```python
from build123d import *

# Parameters (mm, degrees)
SKETCH1_W           = 65
SKETCH1_H           = 68
BOSS_EXTRUDE1_DEPTH = 20
FILLET1_R           = 5
FILLET2_R           = 2
CUT_EXTRUDE1_DEPTH  = 2
FILLET3_R           = 0.5
SKETCH3_W           = 3
SKETCH3_H           = 3
BOSS_EXTRUDE2_DEPTH = 4
FILLET4_R           = 0.2


with BuildPart() as part:
    # Sketch1 → Boss-Extrude1 (new body)
    with BuildSketch(Plane(origin=(0, 0, 0), x_dir=(1, 0, 0), z_dir=(0, 1, 0))):
        Rectangle(SKETCH1_W, SKETCH1_H)
    extrude(amount=BOSS_EXTRUDE1_DEPTH)

    # Fillet1
    fillet1_edges = [part.edges().sort_by_distance(p)[0] for p in [
        (-32.5, 20, 0),
        (32.5, 20, 0),
        (-32.5, 0, 0),
        (32.5, 0, 0),
    ]]
    fillet(fillet1_edges, radius=FILLET1_R)

    # Fillet2
    fillet2_edges = [part.edges().sort_by_distance(p)[0] for p in [
        (-32.5, 10, 34),
        (-32.5, 10, -34),
        (0, 0, 34),
        (32.5, 10, 34),
        (0, 20, 34),
        (31.035533906, 18.535533906, 34),
        (31.035533906, 1.464466094, 34),
        (-31.035533906, 18.535533906, 34),
        (-31.035533906, 1.464466094, 34),
        (0, 0, -34),
        (0, 20, -34),
        (32.5, 10, -34),
        (31.035533906, 18.535533906, -34),
        (31.035533906, 1.464466094, -34),
        (-31.035533906, 18.535533906, -34),
        (-31.035533906, 1.464466094, -34),
    ]]
    fillet(fillet2_edges, radius=FILLET2_R)

    # Sketch2 → Cut-Extrude1 (cut)
    with BuildSketch(Plane(origin=(0, 20, 0), x_dir=(1, 0, 0), z_dir=(0, 1, 0))):
        with BuildLine():
            Line((-26.022422588, -26.349516296), (-18.022422588, -26.349516296))
            ThreePointArc((-18.022422588, -26.349516296), (-17.315315807, -26.642409515), (-17.022422588, -27.349516296))
            Line((-17.022422588, -27.349516296), (-17.022422588, -29.349516296))
            ThreePointArc((-17.022422588, -29.349516296), (-17.315315807, -30.056623077), (-18.022422588, -30.349516296))
            Line((-18.022422588, -30.349516296), (-26.022422588, -30.349516296))
            ThreePointArc((-26.022422588, -30.349516296), (-26.729529369, -30.056623077), (-27.022422588, -29.349516296))
            Line((-27.022422588, -29.349516296), (-27.022422588, -27.349516296))
            ThreePointArc((-27.022422588, -27.349516296), (-26.729529369, -26.642409515), (-26.022422588, -26.349516296))
        make_face()
    extrude(amount=-CUT_EXTRUDE1_DEPTH, mode=Mode.SUBTRACT)

    # Fillet3
    fillet3_edges = [part.edges().sort_by_distance(p)[0] for p in [
        (-26.729529369, 20, 26.642409515),
        (-27.022422588, 20, 28.349516296),
        (-26.729529369, 20, 30.056623077),
        (-22.022422588, 20, 30.349516296),
        (-17.315315807, 20, 30.056623077),
        (-17.022422588, 20, 28.349516296),
        (-17.315315807, 20, 26.642409515),
        (-22.022422588, 20, 26.349516296),
    ]]
    fillet(fillet3_edges, radius=FILLET3_R)

    # Sketch3 → Boss-Extrude2 (add)
    with BuildSketch(Plane(origin=(0, 18, 0), x_dir=(1, 0, 0), z_dir=(0, 1, 0))):
        with Locations((-20.584643458, -28.349516296)):
            Rectangle(SKETCH3_W, SKETCH3_H)
    extrude(amount=BOSS_EXTRUDE2_DEPTH)

    # Fillet4
    fillet4_edges = [part.edges().sort_by_distance(p)[0] for p in [
        (-19.084643458, 18, 28.349516296),
        (-19.084643458, 20, 29.849516296),
        (-20.584643458, 18, 26.849516296),
        (-19.084643458, 20, 26.849516296),
        (-22.084643458, 18, 28.349516296),
        (-22.084643458, 20, 26.849516296),
        (-20.584643458, 18, 29.849516296),
        (-22.084643458, 20, 29.849516296),
        (-19.084643458, 22, 28.349516296),
        (-20.584643458, 22, 26.849516296),
        (-22.084643458, 22, 28.349516296),
        (-20.584643458, 22, 29.849516296),
    ]]
    fillet(fillet4_edges, radius=FILLET4_R)


solid = part.part
```
Can you work these out from the model? Positions are in its coordinate system, mm. A direction names the side the tool comes from. Coordinates: 2 decimals unless noted, no trailing zeros. Loops run counter-clockwise (first coordinate to the right, second up) from the corner with the lowest first, then second, coordinate; pieces in that order, holes last.
Item 1: Which directions (+Z, -Z, +X, -X, +Y, -Y) give clear straight access to the entire face, cutting with the end or side of a thin tool? Please do faces 4 (the face through (-31.07, 18.5, -0.45)), 5 (the face through (-21, 20, 29.85)).
Answers below:
face 4: +Z, -Z, -X, +Y
face 5: +Y
Item 2: Suppose I cut it at B-B (z = 22.5). Please give me the cut outline in (x, y), then the cut area to 3 significant figures.
Answers below:
outline: (-32.5, 5) arc R5 ccw to (-27.5, 0) - (27.5, 0) arc R5 ccw to (32.5, 5) - (32.5, 15) arc R5 ccw to (27.5, 20) - (-27.5, 20) arc R5 ccw to (-32.5, 15) - close
area: 1,280 mm2
Item 3: If we mould it in two halves opening along X, with no side actions, what happens to faces 1 (the face through (-0.39, 0.57, 33.4)), 2 (the face through (-21, 20, 26.85)), 3 (the face through (-32.5, 10, 0))? For each: released by +X, released by -X, zero draft, split by the parting line, or undercut.
Answers below:
face 1: zero draft
face 2: undercut
face 3: released by -X
Item 4: Suppose I cut it at A-A (x = 7). Please give me the cut outline in (y, z).
Answers below:
outline: (0, -32) arc R2 ccw to (2, -34) - (18, -34) arc R2 ccw to (20, -32) - (20, 32) arc R2 ccw to (18, 34) - (2, 34) arc R2 ccw to (0, 32) - close
Item 5: Please list where these lines run through material, in increasing order: L1, parallel to Y at x = -23.5, z = 24.5; L2, parallel to X at y = 19, z = -3; L3, parallel to Z at x = 4, y = 1.75.
Answers below:
L1: y = 0 to 20
L2: x = -30.5 to 30.5
L3: z = -33.98 to 33.98
Item 6: I'm going to push flat-ended pins straight in: pin 1 (2 mm diameter, centred on y = 19.5, z = 29, fed in from -X); pin 2 (2 mm diameter, centred on x = -20, y = 20, fed in from -Z); pin 3 (1.2 mm diameter, centred on x = -22.5, y = 19, fed in from +Z). Where does each tip first touch, or does it pass through?
Answers below:
pin 1: stops at x = -31.07
pin 2: stops at z = -33.73
pin 3: stops at z = 33.96
